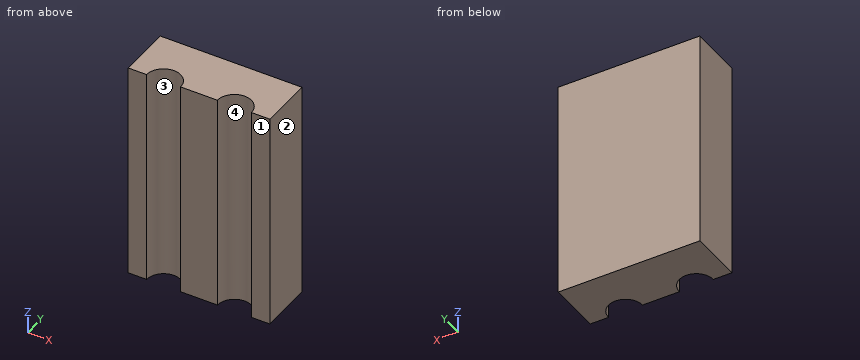
```python
from build123d import *

# Parameters (mm, degrees)
F0_W     = 40
F0_H     = 15
F1_DEPTH = 62
F3_DEPTH = 62.001


with BuildPart() as f1:
    # F0 (on Top) → F1 (new body)
    with BuildSketch(Plane.XY):
        with Locations((20, 7.5)):
            Rectangle(F0_W, F0_H)
    extrude(amount=F1_DEPTH)

    # F2 (on face) → F3 (cut, through all)
    with BuildSketch(Plane(origin=(0, 0, 0), x_dir=(1, 0, 0), z_dir=(0, 0, -1))):
        with BuildLine():
            Line((14.8, 0), (5.2, 0))
            ThreePointArc((5.2, 0), (10, -4.8), (14.8, 0))
        make_face()
        with BuildLine():
            Line((34.8, 0), (25.2, 0))
            ThreePointArc((25.2, 0), (30, -4.8), (34.8, 0))
        make_face()
    extrude(amount=-F3_DEPTH, mode=Mode.SUBTRACT)


solid = f1.part
```
Can you work these out from the model? Positions are in its coordinate system, mm. Face numbers are marked on the shaded views. Coordinates: 2 decimals unless noted, no trailing zeros. Loops run counter-clockwise (first coordinate to the right, second up) from the corner with the lowest first, then second, coordinate; pieces in that order, holes last.
Item 1: Suppose I cut it at D-D (x = 14). Please give me the cut outline in (y, z), then the cut area to 3 significant figures.
Answers below:
outline: (2.65, 0) - (15, 0) - (15, 62) - (2.65, 62) - close
area: 765 mm2
Item 2: If we mould it in two halves opening along X, with no side actions, what happens to the marked faces 1, 2, 3 and 4? For each: released by +X, released by -X, zero draft, split by the parting line, or undercut.
Answers below:
face 1: zero draft
face 2: released by +X
face 3: undercut
face 4: undercut
Item 3: Please list where these lines run through material, in increasing order: L1, parallel to X at y = 1.25, z = 34.5; L2, parallel to X at y = 3.25, z = 23.5; L3, parallel to Y at x = 30, z = 27.
Answers below:
L1: x = 0 to 5.37, 14.63 to 25.37, 34.63 to 40
L2: x = 0 to 6.47, 13.53 to 26.47, 33.53 to 40
L3: y = 4.8 to 15
Item 4: Suppose I cut it at A-A (y = 3). Please give me the cut outline in (x, z).
Answers below:
outline: (0, 0) - (6.25, 0) - (6.25, 62) - (0, 62) - close; (13.75, 0) - (26.25, 0) - (26.25, 62) - (13.75, 62) - close; (33.75, 0) - (40, 0) - (40, 62) - (33.75, 62) - close
Item 5: Suppose I cut it at B-B (z = 36). Please give me the cut outline in (x, y), then the cut area to 3 significant figures.
Answers below:
outline: (0, 0) - (5.2, 0) arc R4.8 cw to (14.8, 0) - (25.2, 0) arc R4.8 cw to (34.8, 0) - (40, 0) - (40, 15) - (0, 15) - close
area: 528 mm2
Item 6: Suppose I cut it at C-C (x = 10). Please give me the cut outline in (y, z), then the cut area to 3 significant figures.
Answers below:
outline: (4.8, 0) - (15, 0) - (15, 62) - (4.8, 62) - close
area: 632 mm2
Item 7: I'm going to push flat-ended pins straight in: pin 1 (3 mm diameter, centred on y = 9, z = 41, fed in from -X); pin 2 (3 mm diameter, centred on x = 28, z = 44.5, fed in from -Y). Where does each tip first touch, or does it pass through?
Answers below:
pin 1: stops at x = 0
pin 2: stops at y = 3.28
